Read the model definition and answer for the solid it produces. Units are mm, in the model's axes. A direction names the side the tool comes from. Coordinates: 2 decimals unless noted, no trailing zeros. Order: outer loops, then holes, each group sorted by start corner. A loop starts at its lowest first (then second) coordinate and runs counter-clockwise, first axis right, second up. Notation, with made-up numbers: (73.5, 73.25) -> (95.5, 73.25) arc R18 ccw to (95.5, 92.25) -> close; hole circle Ø7 at (69.25, 10.25). An arc over 180 degrees is marked (long way). Answer as a JSON object with one key per item and string values. Group by question number.
1) Consider L1, parallel to X at y = 5.25, z = 0; L2, parallel to X at y = 8.5, z = 10.5; L3, parallel to X at y = 0.5, z = 14.5. Determine where each line is inside the solid, lowest interval first.
2) Section D-D on x = 7 is taken. Determine the outline of the cut face in (y, z).
3) Section C-C on z = -7 is taken. Determine the outline of the cut face in (x, y).
4) Given pin 1 (2.5 mm diameter, centred on x = -28.5, y = 3.5, fed in from +Z); pin 2 (1.5 mm diameter, centred on x = 20.5, y = 1, fed in from +Z); pin 3 (2.5 mm diameter, centred on y = 7, z = 0.5, fed in from -X), each flat-ended and moving along its own axis, determine where each tip first touches the part or whether it passes through.
5) Determine the mould class of faces 1 (the cylindrical face through (7.89, -1.01, 0.12)), 2 (the flat face through (-14.39, 4.93, 14.68)), 3 (the cylindrical face through (19.276, 4.93, -18.906)), 4 (the flat face through (28, 5, 2.5)) for opening direction Z: released by +Z, released by -Z, zero draft, split by the parting line, or undercut.
6) Section B-B on y = 3.5 is taken. Determine the outline of the cut face in (x, z), and give its area (3 significant figures).
7) A tool of negligible diameter and unlimited length cuts with its end or side. For faces 5 (the cylindrical face through (-19.276, 4.93, 18.906)), 6 (the cylindrical face through (-18.906, 4.93, -19.276)), 7 (the cylindrical face through (0.828, 4.93, -24.986)), 8 (the flat face through (29.8, 5, 0)), from which of +Z, -Z, +X, -X, +Y, -Y can it reach the whole face along a straight path? Write none if from no direction.
8) Section A-A on x = 0 is taken. Determine the outline of the cut face in (y, z), and give its area (3 significant figures).
from build123d import *

# Parameters (mm, degrees)
SKETCH1_R           = 27
SKETCH1_R_2         = 14
BOSS_EXTRUDE1_DEPTH = 10
SKETCH2_R           = 32.5
BOSS_EXTRUDE2_DEPTH = 2
SKETCH3_W           = 5
SKETCH3_H           = 4.39677325
SKETCH3_W_2         = 4.39677325
SKETCH3_H_2         = 5
BOSS_EXTRUDE3_DEPTH = 10
CUT_EXTRUDE1_REACH  = 49.503
SKETCH4_R           = 0.9


with BuildPart() as part:
    # Sketch1 → Boss-Extrude1 (new body)
    with BuildSketch(Plane(origin=(0, 0, 0), x_dir=(1, 0, 0), z_dir=(0, 1, 0))):
        with Locations(Location((0, 0, 0), (0, 0, 270))):
            Circle(SKETCH1_R)
        with Locations(Location((0, 0, 0), (0, 0, 270))):
            Circle(SKETCH1_R_2, mode=Mode.SUBTRACT)
        with BuildLine():
            Line((-17.5, -17.853571071), (-11.2, -11.426285486))
            ThreePointArc((-11.2, -11.426285486), (0, 16), (11.2, -11.426285486))
            Line((11.2, -11.426285486), (17.5, -17.853571071))
            ThreePointArc((17.5, -17.853571071), (0, 25), (-17.5, -17.853571071))
        make_face(mode=Mode.SUBTRACT)
    extrude(amount=BOSS_EXTRUDE1_DEPTH)

    # Sketch2 → Boss-Extrude2 (add)
    with BuildSketch(Plane.XZ):
        with Locations(Location((0, 0, 0), (0, 0, 270))):
            Circle(SKETCH2_R)
    extrude(amount=BOSS_EXTRUDE2_DEPTH)

    # Sketch3 → Boss-Extrude3 (add)
    with BuildSketch(Plane(origin=(0, 0, 0), x_dir=(1, 0, 0), z_dir=(0, 1, 0))):
        with Locations((0, 27.601613375)):
            Rectangle(SKETCH3_W, SKETCH3_H)
        with Locations((27.601613375, 0)):
            Rectangle(SKETCH3_W_2, SKETCH3_H_2)
        with Locations((0, -27.601613375)):
            Rectangle(SKETCH3_W, SKETCH3_H)
        with Locations((-27.601613375, 0)):
            Rectangle(SKETCH3_W_2, SKETCH3_H_2)
    extrude(amount=BOSS_EXTRUDE3_DEPTH)

    # Sketch4 → Cut-Extrude1 (cut, up to next)
    with BuildSketch(Plane.XZ.offset(2), mode=Mode.PRIVATE) as cut_extrude1_sk1:
        with Locations(Location((0, -7, 0), (0, 0, 270))):
            Circle(SKETCH4_R)
    cut_extrude1_tool1 = extrude(cut_extrude1_sk1.sketch, amount=-CUT_EXTRUDE1_REACH, mode=Mode.PRIVATE) & part.part
    # Sketch4 → Cut-Extrude1 (cut, up to next)
    with BuildSketch(Plane.XZ.offset(2), mode=Mode.PRIVATE) as cut_extrude1_sk2:
        with Locations(Location((-7, 0, 0), (0, 0, 270))):
            Circle(SKETCH4_R)
    cut_extrude1_tool2 = extrude(cut_extrude1_sk2.sketch, amount=-CUT_EXTRUDE1_REACH, mode=Mode.PRIVATE) & part.part
    # Sketch4 → Cut-Extrude1 (cut, up to next)
    with BuildSketch(Plane.XZ.offset(2), mode=Mode.PRIVATE) as cut_extrude1_sk3:
        with Locations(Location((0, 7, 0), (0, 0, 270))):
            Circle(SKETCH4_R)
    cut_extrude1_tool3 = extrude(cut_extrude1_sk3.sketch, amount=-CUT_EXTRUDE1_REACH, mode=Mode.PRIVATE) & part.part
    # Sketch4 → Cut-Extrude1 (cut, up to next)
    with BuildSketch(Plane.XZ.offset(2), mode=Mode.PRIVATE) as cut_extrude1_sk4:
        with Locations(Location((7, 0, 0), (0, 0, 270))):
            Circle(SKETCH4_R)
    cut_extrude1_tool4 = extrude(cut_extrude1_sk4.sketch, amount=-CUT_EXTRUDE1_REACH, mode=Mode.PRIVATE) & part.part
    add(cut_extrude1_tool1.solids().sort_by_distance((0, -2, -7))[0], mode=Mode.SUBTRACT)
    add(cut_extrude1_tool2.solids().sort_by_distance((-7, -2, 0))[0], mode=Mode.SUBTRACT)
    add(cut_extrude1_tool3.solids().sort_by_distance((0, -2, 7))[0], mode=Mode.SUBTRACT)
    add(cut_extrude1_tool4.solids().sort_by_distance((7, -2, 0))[0], mode=Mode.SUBTRACT)


solid = part.part
Worked answers:
{
 "1": {"L1": "x = -29.8 to -25, -16 to -14, 14 to 16, 25 to 29.8", "L2": "x = -24.87 to -22.69, -12.07 to -9.26, 9.26 to 12.07, 22.69 to 24.87", "L3": "x = -22.78 to -20.37, -14.21 to 14.21, 20.37 to 22.78"},
 "2": {"outline": "(-2, -31.74) -> (0, -31.74) -> (0, -26.08) -> (10, -26.08) -> (10, -24) -> (0, -24) -> (0, -14.39) -> (10, -14.39) -> (10, -12.12) -> (0, -12.12) -> (0, -0.9) -> (-2, -0.9) -> close; (-2, 0.9) -> (0, 0.9) -> (0, 12.12) -> (10, 12.12) -> (10, 26.08) -> (0, 26.08) -> (0, 31.74) -> (-2, 31.74) -> close"},
 "3": {"outline": "(-31.74, -2) -> (-0.9, -2) -> (-0.9, 0) -> (-12.12, 0) -> (-12.12, 10) -> (-14.39, 10) -> (-14.39, 0) -> (-24, 0) -> (-24, 10) -> (-26.08, 10) -> (-26.08, 0) -> (-31.74, 0) -> close; (0.9, -2) -> (31.74, -2) -> (31.74, 0) -> (26.08, 0) -> (26.08, 10) -> (24, 10) -> (24, 0) -> (14.39, 0) -> (14.39, 10) -> (12.12, 10) -> (12.12, 0) -> (0.9, 0) -> close"},
 "4": {"pin 1": "stops at z = 2.5", "pin 2": "stops at z = 18.41", "pin 3": "stops at x = -29.8"},
 "5": {"face 1": "undercut", "face 2": "undercut", "face 3": "released by -Z", "face 4": "released by +Z"},
 "6": {"outline": "(-29.8, -2.5) -> (-26.88, -2.5) arc R27 ccw to (-2.5, -26.88) -> (-2.5, -29.8) -> (2.5, -29.8) -> (2.5, -26.88) arc R27 ccw to (26.88, -2.5) -> (29.8, -2.5) -> (29.8, 2.5) -> (26.88, 2.5) arc R27 ccw to (2.5, 26.88) -> (2.5, 29.8) -> (-2.5, 29.8) -> (-2.5, 26.88) arc R27 ccw to (-26.88, 2.5) -> (-29.8, 2.5) -> close; hole (-17.5, 17.85) arc R25 ccw (long way) to (17.5, 17.85) -> (11.2, 11.43) arc R16 cw (long way) to (-11.2, 11.43) -> close; hole circle Ø28 at (0, 0)", "area": "858 mm²"},
 "7": {"face 5": "+Z, -X, +Y", "face 6": "-Z, -X, +Y", "face 7": "+Y", "face 8": "+Z, -Z, +X, +Y"},
 "8": {"outline": "(-2, -32.5) -> (0, -32.5) -> (0, -29.8) -> (10, -29.8) -> (10, -25) -> (0, -25) -> (0, -16) -> (10, -16) -> (10, -14) -> (0, -14) -> (0, -7.9) -> (-2, -7.9) -> close; (-2, -6.1) -> (0, -6.1) -> (0, 6.1) -> (-2, 6.1) -> close; (-2, 7.9) -> (0, 7.9) -> (0, 14) -> (10, 14) -> (10, 29.8) -> (0, 29.8) -> (0, 32.5) -> (-2, 32.5) -> close", "area": "349 mm²"}
}
